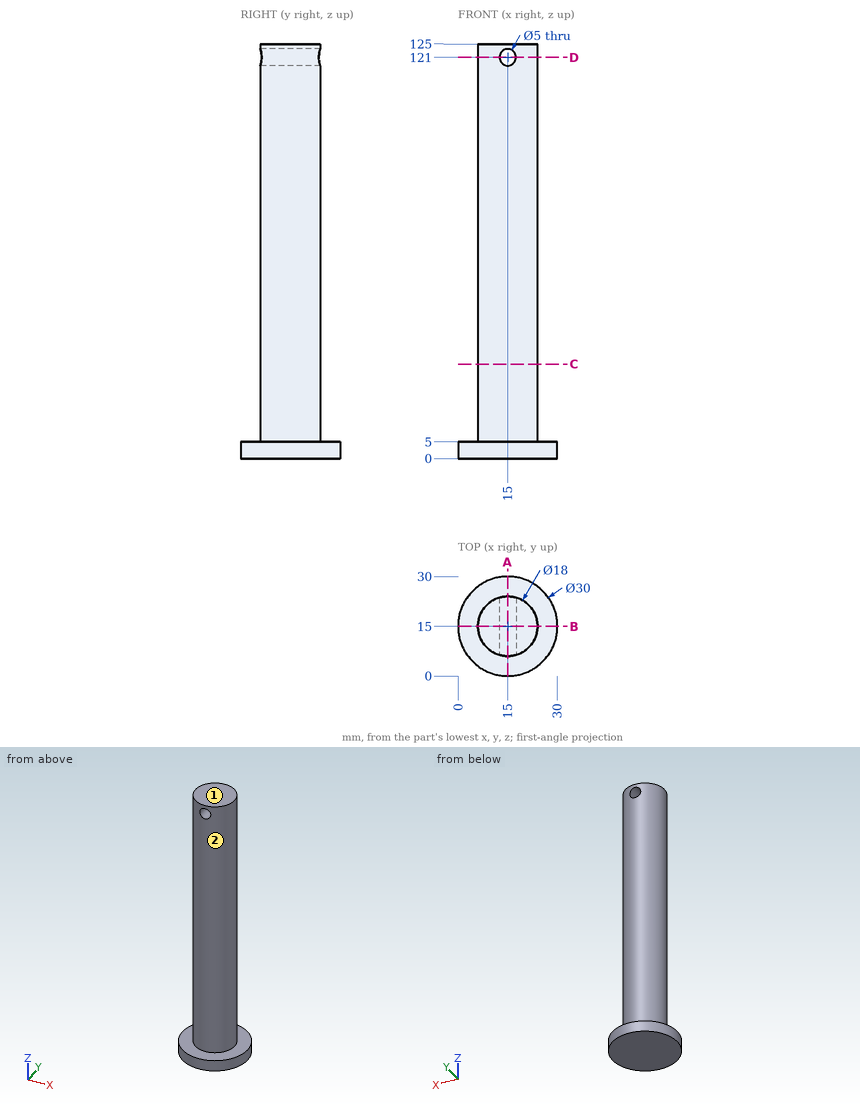
For this review, use the dimensioned drawing (mm, ordinates from the lowest corner) and the shaded views. A direction names the side the tool comes from. Round coordinates to 2 decimals unless told otherwise and drop trailing zeros. Order: outer loops, then holes, each group sorted by start corner. A loop starts at its lowest first (then second) coordinate and runs counter-clockwise, first axis right, second up. Notation, with made-up numbers: M -2,68.25 L 13,68.25 A15 cw 13,94.25 Z; hole C 7,72 d3. An arc over 180 degrees is marked long. Write each question's results on one line, items separated by ' | '. Start each with the question number.
1. Add section B-B (y = 15). State the section outline as (x, z) points.
2. To check wall thickness, follow L1, parallel to Z at x = 15, y = 14.75; L2, parallel to X at y = 17.25, z = 121; L3, parallel to Z at x = 13.5, y = 2.5. State the ranges of each line that lie inside material, in increasing order. Write a range as [from, to].
3. Clearance check with flat-ended pins moving along their axes: pin 1 Ø4 at (y, z) = (17.5, 36.5) entering from -X; pin 2 Ø5 at (y, z) = (19.5, 17.5) entering from +X; pin 3 Ø8 at (y, z) = (11.5, 83.5) entering from +X; pin 4 Ø8 at (x, y) = (6, 9) entering from -Z. State where each tip first meets the part, or that it passes through.
4. Add section C-C (z = 28.5). State the section outline as (x, y) points.
5. Add section D-D (z = 121). State the section outline as (x, y) points, then the cut area to 3 significant figures.
6. Add section A-A (x = 15). State the section outline as (y, z) points.
7. Tool access review of the marked faces 1 and 2: name each direction out of +Z, -Z, +X, -X, +Y, -Y from which nothing blocks a thin tool from reaching the whole face with its end or side.
Output values:
1) outline: M 0,0 L 30,0 L 30,5 L 24,5 L 24,125 L 6,125 L 6,5 L 0,5 Z; hole C 15,121 d5
2) L1: [0, 118.5], [123.5, 125] | L2: [6.29, 12.5], [17.5, 23.71] | L3: [0, 5]
3) pin 1: x = 6.01 | pin 2: x = 23.77 | pin 3: x = 24 | pin 4: z = 0
4) outline: C 15,15 d18
5) outline: M 12.5,6.35 L 12.5,23.65 A9 ccw Z; M 17.5,6.35 A9 ccw 17.5,23.65 Z | area: 166 mm^2
6) outline: M 0,0 L 30,0 L 30,5 L 24,5 L 24,118.5 L 6,118.5 L 6,5 L 0,5 Z; M 6,123.5 L 24,123.5 L 24,125 L 6,125 Z
7) face 1: +Z, +X, -X, +Y, -Y | face 2: +Z
